Autodesk Inventor part; units mm, degrees
ref_plane "YZ Plane" through (0, 0, 0) normal (1, 0, 0) x (0, 1, 0)
ref_plane "XZ Plane" through (0, 0, 0) normal (0, 1, 0) x (-1, 0, 0)
ref_plane "XY Plane" through (0, 0, 0) normal (0, 0, 1) x (1, 0, 0)
sketch "Skizze1" plane through (0, 0, 0) normal (0, 0, 1) x (1, 0, 0)
  line L0 (0, 0) -> (-39.55, 0)
  line L1 (-39.55, 0) -> (-39.55, 2)
  line L2 (-39.55, 2) -> (-33.35, 2)
  line L3 (-33.35, 2) -> (-33.35, 2.5)
  line L4 (-33.35, 2.5) -> (-33.05, 2.5)
  line L5 (-33.05, 2.5) -> (-33.05, 4)
  line L6 (-33.05, 4) -> (-32.05, 4)
  line L7 (-32.05, 4) -> (-32.05, 3)
  line L8 (0, 0) -> (0, 3) construction
  line L9 (0, 3) -> (-32.05, 3)
  line L10 (0, 0) -> (39.55, 0)
  line L11 (39.55, 0) -> (39.55, 2)
  line L12 (39.55, 2) -> (33.3, 2)
  line L13 (33.3, 2) -> (33.05, 2)
  line L14 (33.05, 2) -> (25.05, 2)
  line L15 (0, 3) -> (25.05, 3)
  line L16 (25.05, 3) -> (25.05, 2)
  line L17 (-39.55, 2) -> (-39.65, 2)
  line L18 (-39.65, 2) -> (-39.65, 1.85)
  line L19 (-39.65, 1.85) -> (-40.15, 1.85)
  line L20 (-40.15, 1.85) -> (-40.15, 2)
  line L21 (-40.15, 2) -> (-40.65, 2)
  line L22 (-40.65, 2) -> (-40.65, 0)
  line L23 (-40.65, 0) -> (-39.55, 0)
  line L24 (39.55, 2) -> (39.65, 2)
  line L25 (39.65, 2) -> (39.65, 1.85)
  line L26 (39.65, 1.85) -> (40.15, 1.85)
  line L27 (40.15, 1.85) -> (40.15, 2)
  line L28 (40.15, 2) -> (40.65, 2)
  line L29 (40.65, 2) -> (40.65, 0)
  line L30 (40.65, 0) -> (39.55, 0)
  dimension "d0" = 39.55
  dimension "d1" = 2
  dimension "d2" = 6.2
  dimension "d3" = 0.5
  dimension "d4" = 0.3
  dimension "d5" = 1.5
  dimension "d6" = 1
  dimension "d7" = 3
  dimension "d8" = 32.05
  dimension "d9" = 39.55
  dimension "d10" = 2
  dimension "d13" = 0.25
  dimension "d14" = 8
  dimension "d16" = 25.05
  dimension "d17" = 0.1
  dimension "d18" = 0.15
  dimension "d19" = 0.5
  dimension "d20" = 0.5
  dimension "d21" = 0.1
  dimension "d22" = 0.15
  dimension "d23" = 0.5
  dimension "d24" = 0.5
revolve "Umdrehung1" add sketch "Skizze1" angle 360 about axis through (0, 0, 0) along (-1, 0, 0)
sketch "Skizze2" plane through (0, 0, 0) normal (0, 1, 0) x (-1, 0, 0)
  line L0 (-25.05, -3) -> (-25.05, 3)
  line L1 (-25.05, 0) -> (-27.3, 0)
  point P0 (0, 0)
  dimension "d26" = 2.25
hole "Bohrung1" at (27.3, 0, 0) direction (0, -1, 0) diameter 2.459 depth 8.8
hole "Bohrung2" at (27.3, 0, 0) direction (0, 1, 0) diameter 2.459 depth 8.8
chamfer "Fasen1" distance 0.1 angle 45 1 edges at (25.05, -3, 0)
properties part number "DribblerWelle"
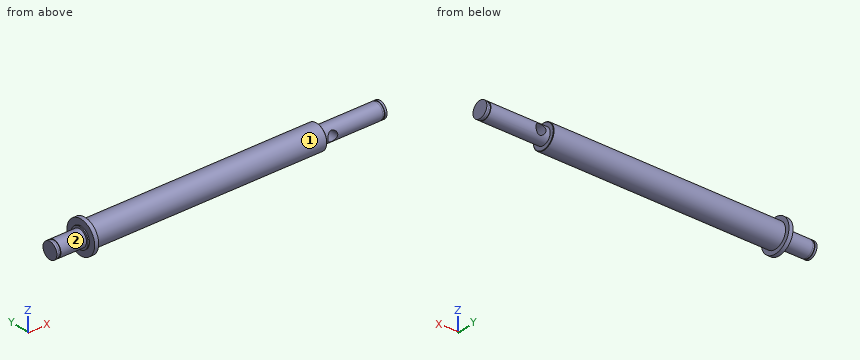
Can you work these out from the model? Positions are in its coordinate system, mm. Face numbers are marked on the shaded views. A direction names the side the tool comes from. Coordinates: 2 decimals unless noted, no trailing zeros. Write each loop counter-clockwise with the first axis right and the second up, starting at its lowest first coordinate (ties: lowest second). Pieces come first, ordered by that corner, then holes.
Q1. For P1, Ø2, axis at x = 27.3, z = 0, coming from the -Y side; P2, Ø4, axis at x = -2, z = -2, coming from the -Y side; P3, Ø1.5, axis at y = 1.5, z = 3, coming from the -X side; P4, Ø3, axis at x = 11, z = -0.5, coming from the +Y side, each with a flat end and sliding along its axis, tell me the tip position at first contact or that it passes through.
Results found:
P1: passes through
P2: stops at y = -3
P3: stops at x = -33.05
P4: stops at y = 3
Q2. Please list where these lines run through material, in increasing order: L1, parallel to Z at x = 27.3, y = 0.2; L2, parallel to X at y = -0.4, z = 0; L3, parallel to Z at x = 35, y = 0.25.
Results found:
L1: z = -1.99 to -1.23, 1.23 to 1.99
L2: x = -40.65 to 26.07, 28.53 to 40.65
L3: z = -1.98 to 1.98
Q3. Imagine slicing it at B-B, the plane x = -15.5. List the corners of the cut face in (y, z) for me.
Results found:
outline: circle Ø6 at (0, 0)
Q4. Which directions (+Z, -Z, +X, -X, +Y, -Y) give clear straight access to the entire face, cutting with the end or side of a thin tool? Please do the marked faces 1 and 2.
Results found:
face 1: +X
face 2: -X
Q5. Imagine slicing it at A-A, the plane x = 27.3. List the corners of the cut face in (y, z) for me, plus the area to 3 significant figures.
Results found:
outline: (-1.58, -1.23) arc R2 ccw to (1.58, -1.23) - close; (-1.58, 1.23) - (1.58, 1.23) arc R2 ccw to start
area: 3.39 mm2
